Geometry: final body of the model. Coordinates: model frame, mm. Face numbers are marked on the shaded views. A direction names the side the tool comes from. Coordinates: 2 decimals unless noted, no trailing zeros. Order: outer loops, then holes, each group sorted by start corner. A loop starts at its lowest first (then second) coordinate and runs counter-clockwise, first axis right, second up. Notation, with made-up numbers: (-25.75, -14.5) -> (-9.75, -14.5) arc R23 ccw to (-9.75, 24.5) -> close; hole circle Ø11 at (-10, 52). An arc over 180 degrees is marked (long way). Answer in a Markdown table with one row per item. Add a question column.
1) Ray query, line 1 (X direction, y = 8.5, z = -38.5); line 2 (Z direction, x = 11, y = -2.75); line 3 (Y direction, x = 41.5, z = -17.5). Return the intervals inside material, ascending. Write a range as from..to.
2) Section query C-C on z = -39. Return the cut outline in (x, y).
3) Section query B-B on y = -1.5. Return the cut outline in (x, z), then the cut area to 3 significant figures.
4) Section query A-A on x = 33. Return the cut outline in (y, z).
5) Section query D-D on x = 13.5. Return the cut outline in (y, z).
6) Pull-direction query (X, two-part tool) for the marked faces 1, 2, 3 and 4; classes: +X half, -X half, draft (parallel to the pull), parting line (faces both ways), or undercut.
7) Contact query for flat-ended pins moving along their axis: P1, Ø1.5, axis at x = 49, y = 7, coming from the -Z side; P2, Ø1.6, axis at y = 11, z = -1, coming from the +X side; P3, Ø0.6, axis at y = -2.5, z = -1, coming from the -X side. Output: stop coordinate, or through.
8) Set-up query: the marked faces 5, 6 and 7. Return all of +Z, -Z, +X, -X, +Y, -Y with unobstructed straight access to the full face (end or side cutting, diameter ignored); none if empty.
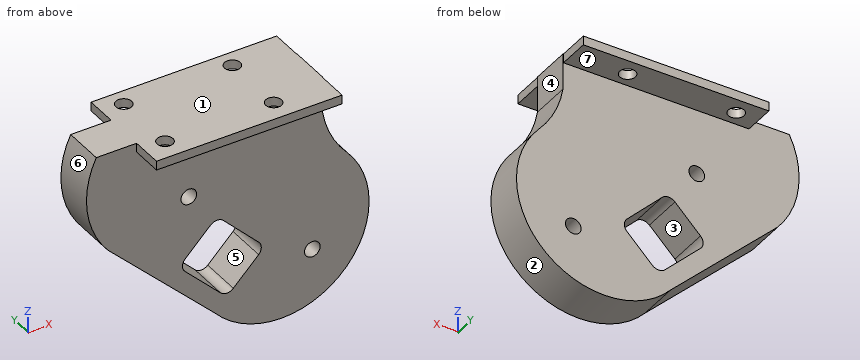
```python
from build123d import *

# Parameters (mm, degrees)
BOSS_EXTRUDE1_DEPTH = 9
SKETCH2_W           = 41
SKETCH2_H           = 7
BOSS_EXTRUDE2_DEPTH = 2
SKETCH3_R           = 1.75
CUT_EXTRUDE1_DEPTH  = 2
SKETCH5_R           = 1.725
CUT_EXTRUDE4_DEPTH  = 9
CUT_EXTRUDE5_DEPTH  = 9
FILLET1_R           = 2


with BuildPart() as part:
    # Sketch1 → Boss-Extrude1 (new body)
    with BuildSketch(Plane(origin=(0, 0, 0), x_dir=(1, 0, 0), z_dir=(0, 1, 0))):
        with BuildLine():
            Line((0, 0), (50, 0))
            Line((50, 0), (50, 8))
            ThreePointArc((50, 8), (51.881677867, 13.952299325), (55.397568431, 19.110699502))
            ThreePointArc((55.397568431, 19.110699502), (53.716316301, 46.611180772), (26.21583503, 44.929928642))
            Line((26.21583503, 44.929928642), (2.535645118, 21.946269105))
            ThreePointArc((2.535645118, 21.946269105), (-2.034097015, 11.354634306), (0, 0))
        make_face()
    extrude(amount=BOSS_EXTRUDE1_DEPTH)

    # Sketch2 → Boss-Extrude2 (add)
    with BuildSketch(Plane.XY):
        with Locations((29.413010925, -3.5)):
            Rectangle(SKETCH2_W, SKETCH2_H)
        with Locations((29.413010925, 12.5)):
            Rectangle(SKETCH2_W, SKETCH2_H)
    extrude(amount=-BOSS_EXTRUDE2_DEPTH)

    # Sketch3 → Cut-Extrude1 (cut)
    with BuildSketch(Plane(origin=(0, 0, -2), x_dir=(-1, 0, 0), z_dir=(0, 0, -1))):
        with Locations((-13.769448398, -2.263474859)):
            Circle(SKETCH3_R)
        with Locations((-37.769448398, -2.263474859)):
            Circle(SKETCH3_R)
        with Locations((-37.769448398, 12.236525141)):
            Circle(SKETCH3_R)
        with Locations((-13.769448398, 12.236525141)):
            Circle(SKETCH3_R)
    extrude(amount=-CUT_EXTRUDE1_DEPTH, mode=Mode.SUBTRACT)

    # Sketch5 → Cut-Extrude4 (cut)
    with BuildSketch(Plane(origin=(0, 9, 0), x_dir=(1, 0, 0), z_dir=(0, 1, 0))):
        with Locations(Location((20.448484722, 16.392658608, 0), (0, 0, 270))):
            Circle(SKETCH5_R)
        with Locations(Location((47.74101634, 38.304247275, 0), (0, 0, 270))):
            Circle(SKETCH5_R)
    extrude(amount=-CUT_EXTRUDE4_DEPTH, mode=Mode.SUBTRACT)

    # Sketch6 → Cut-Extrude5 (cut)
    with BuildSketch(Plane(origin=(0, 9, 0), x_dir=(1, 0, 0), z_dir=(0, 1, 0))):
        Polygon((18.200821257, 31.659530408), (28.87624988, 42.196855672), (37.292479574, 33.780625977), (26.686102631, 23.174249034), align=None)
    extrude(amount=-CUT_EXTRUDE5_DEPTH, mode=Mode.SUBTRACT)

    # Fillet1
    fillet1_edges = [part.edges().sort_by_distance(p)[0] for p in [
        (18.200821257, 4.5, -31.659530408),
        (26.686102631, 4.5, -23.174249034),
        (37.292479574, 4.5, -33.780625977),
        (28.87624988, 4.5, -42.196855672),
    ]]
    fillet(fillet1_edges, radius=FILLET1_R)


solid = part.part
```
Result:
| question | item | result |
|---|---|---|
| 1 | line 1 | 19.59..25.13, 32.57..46.03, 49.45..59.18 |
| 1 | line 2 | -2..0 |
| 1 | line 3 | 0..9 |
| 2 | outline | (20.11, 0) -> (25.64, 0) -> (25.64, 9) -> (20.11, 9) -> close; (32.07, 0) -> (46.16, 0) -> (46.16, 9) -> (32.07, 9) -> close; (49.32, 0) -> (59, 0) -> (59, 9) -> (49.32, 9) -> close |
| 3 | outline | (8.91, -2) -> (12.19, -2) -> (12.19, 0) -> (8.91, 0) -> close; (15.34, -2) -> (36.19, -2) -> (36.19, 0) -> (15.34, 0) -> close; (39.34, -2) -> (49.91, -2) -> (49.91, 0) -> (39.34, 0) -> close |
| 3 | area | 69.4 mm2 |
| 4 | outline | (-7, -2) -> (0, -2) -> (0, -29.49) -> (9, -29.49) -> (9, -2) -> (16, -2) -> (16, 0) -> (-7, 0) -> close; (0, -49.87) -> (9, -49.87) -> (9, -38.07) -> (0, -38.07) -> close |
| 5 | outline | (-7, -2) -> (-3.99, -2) -> (-3.99, 0) -> (-7, 0) -> close; (-0.53, -2) -> (0, -2) -> (0, -32.59) -> (9, -32.59) -> (9, -2) -> (10.51, -2) -> (10.51, 0) -> (-0.53, 0) -> close; (13.97, -2) -> (16, -2) -> (16, 0) -> (13.97, 0) -> close |
| 6 | face 1 | draft |
| 6 | face 2 | parting line |
| 6 | face 3 | undercut |
| 6 | face 4 | +X half |
| 7 | P1 | z = -50.02 |
| 7 | P2 | x = 49.91 |
| 7 | P3 | x = 8.91 |
| 8 | face 5 | +Y, -Y |
| 8 | face 6 | -X, +Y, -Y |
| 8 | face 7 | -Z, +X, -X, +Y |
